Verification items for the finished model (mm, model axes). Coordinates: 2 decimals unless noted, no trailing zeros. Write each loop counter-clockwise with the first axis right and the second up, starting at its lowest first coordinate (ties: lowest second). Pieces come first, ordered by that corner, then holes. Notation, with made-up numbers: (76.25, -3) -> (113.25, -3) arc R16 ccw to (113.25, 23) -> close; hole circle Ø10 at (59.5, 38). An arc over 180 degrees is marked (long way). Use CSV: the item, a comma, the result in double quotes.
```python
from build123d import *

# Parameters (mm, degrees)
SKETCH1_W           = 25.4
SKETCH1_H           = 50.8
BOSS_EXTRUDE1_DEPTH = 279.4
SHELL1_T            = -3.175
SKETCH3_R           = 2.38125
CUT_EXTRUDE1_DEPTH  = 285.264471927


with BuildPart() as part:
    # Sketch1 → Boss-Extrude1 (new, symmetric)
    with BuildSketch(Plane.XY):
        Rectangle(SKETCH1_W, SKETCH1_H)
    extrude(amount=BOSS_EXTRUDE1_DEPTH, both=True)

    # Shell1
    shell1_openings = [part.faces().sort_by_distance(p)[0] for p in [
        (0, 0, 279.4),
        (0, 0, -279.4),
    ]]
    offset(amount=SHELL1_T, openings=shell1_openings, kind=Kind.INTERSECTION)

    # Sketch3 → Cut-Extrude1 (cut, through all)
    with BuildSketch(Plane(origin=(0, 25.4, 0), x_dir=(1, 0, 0), z_dir=(0, 1, 0))):
        with Locations(Location((0, 266.7, 0), (0, 0, 270))):
            Circle(SKETCH3_R)
        with Locations(Location((0, 241.3, 0), (0, 0, 270))):
            Circle(SKETCH3_R)
        with Locations(Location((0, 215.9, 0), (0, 0, 270))):
            Circle(SKETCH3_R)
        with Locations(Location((0, -215.9, 0), (0, 0, 270))):
            Circle(SKETCH3_R)
        with Locations(Location((0, -241.3, 0), (0, 0, 270))):
            Circle(SKETCH3_R)
        with Locations(Location((0, -266.7, 0), (0, 0, 270))):
            Circle(SKETCH3_R)
        with Locations(Location((0, 66.675, 0), (0, 0, 270))):
            Circle(SKETCH3_R)
        with Locations(Location((0, 15.875, 0), (0, 0, 270))):
            Circle(SKETCH3_R)
        with Locations(Location((0, 41.275, 0), (0, 0, 270))):
            Circle(SKETCH3_R)
        with Locations(Location((0, -85.725, 0), (0, 0, 270))):
            Circle(SKETCH3_R)
        with Locations(Location((0, -60.325, 0), (0, 0, 270))):
            Circle(SKETCH3_R)
        with Locations(Location((0, -111.125, 0), (0, 0, 270))):
            Circle(SKETCH3_R)
        with BuildLine():
            Line((6.35, 279.4), (-12.7, 279.4))
            Line((-12.7, 279.4), (-12.7, 273.05))
            Line((-12.7, 273.05), (0, 273.05))
            ThreePointArc((0, 273.05), (4.490128061, 274.909871939), (6.35, 279.4))
        make_face()
        with BuildLine():
            Line((-12.7, -273.05), (0, -273.05))
            ThreePointArc((0, -273.05), (4.490128061, -274.909871939), (6.35, -279.4))
            Line((6.35, -279.4), (-12.7, -279.4))
            Line((-12.7, -279.4), (-12.7, -273.05))
        make_face()
    extrude(amount=-CUT_EXTRUDE1_DEPTH, mode=Mode.SUBTRACT)


solid = part.part
```
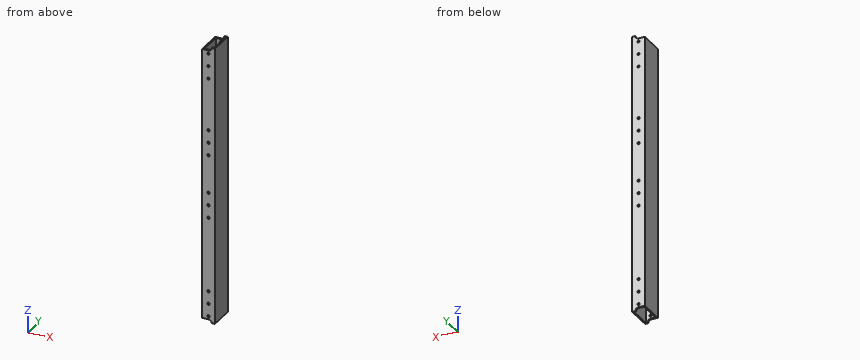
1) Cross-section at A-A (y = -17). Record the boundary of the cut face in (x, z) (3 decimals).
Return value:
outline,"(-12.7, -273.05) -> (-9.525, -273.05) -> (-9.525, 273.05) -> (-12.7, 273.05) -> close; (9.525, -279.4) -> (12.7, -279.4) -> (12.7, 279.4) -> (9.525, 279.4) -> close"
2) Scan lines: L1, parallel to X at y = 11, z = 46.5 (3 decimals); L2, parallel to Y at x = -9.25, z = 250.5 (3 decimals); L3, parallel to X at y = -23, z = -241. Record each from-to range of solid material in increasing order.
Return value:
L1,"-12.7 to -9.525, 9.525 to 12.7"
L2,"-25.4 to -22.225, 22.225 to 25.4"
L3,"-12.7 to -2.36, 2.36 to 12.7"
3) Gauge pin test, flat ends, axial feed: pin 1 (6 mm diameter, centred on x = -9.5, y = -17, fed in from +Z); pin 2 (3 mm diameter, centred on x = 0, z = 60.325, fed in from +Y); pin 3 (3 mm diameter, centred on x = -9.5, y = 14, fed in from -Z). Record the tip position at first contact, or that the pin passes through.
Return value:
pin 1,"z = 273.05"
pin 2,"through"
pin 3,"z = -273.05"
4) Cross-section at B-B (z = -96). Record the boundary of the cut face in (x, y) (3 decimals), plus the area to 3 significant figures.
Return value:
outline,"(-12.7, -25.4) -> (12.7, -25.4) -> (12.7, 25.4) -> (-12.7, 25.4) -> close; hole (-9.525, -22.225) -> (9.525, -22.225) -> (9.525, 22.225) -> (-9.525, 22.225) -> close"
area,"444 mm2"
